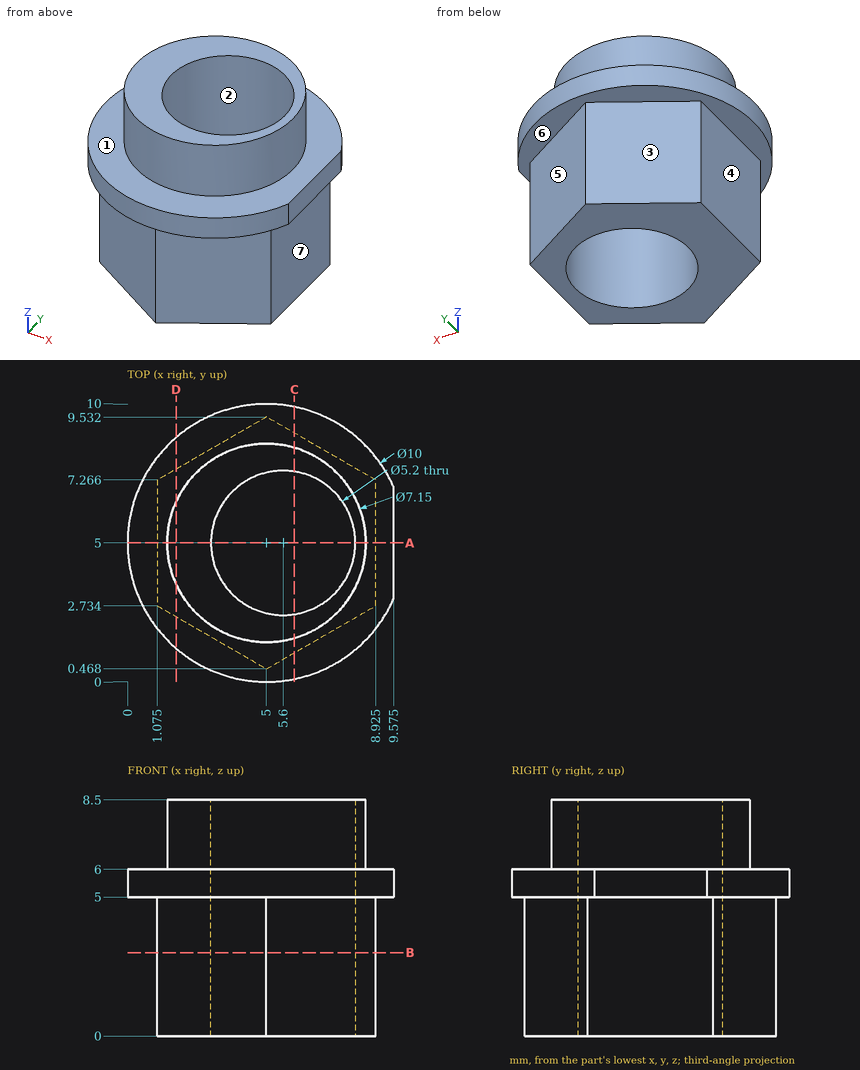
Check sheet for the drawn part. Datum: minimum x, y, z corner. Units: mm. A direction names the side the tool comes from. Round coordinates to 2 decimals unless told otherwise and drop trailing zeros. Order: outer loops, then holes, each group sorted by start corner. A loop starts at its lowest first (then second) coordinate and runs counter-clockwise, first axis right, second up. Notation, with made-up numbers: (36, 49) -> (41, 49) arc R18 cw to (41, 64) -> close; hole circle Ø6 at (78, 45). An arc over 180 degrees is marked (long way). Return JSON: item names as keys, results as strings. Group by question number.
Q1. Section check D-D, the plane x = 1.75. Record the boundary of the cut face in (y, z), plus the area to 3 significant figures.
Q2. Material ranges on probe 1 along Z at (x, y) = (8.5, 6.75); probe 2 along Y at (x, z) = (6, 8.25); probe 3 along X at (y, z) = (6.25, 2.5) (1 decimal), recorded low to high. Write a range as from..to.
Q3. Section check B-B, the plane z = 3. Record the boundary of the cut face in (x, y) (1 decimal), plus the area to 3 significant figures.
Q4. Tool access check on the marked faces 4, 5, 6 and 7. Record the directions out of +Z, -Z, +X, -X, +Y, -Y that give a thin tool (end or side, any length) a straight path to the whole face; none if there is none.
Q5. Section check C-C, the plane x = 6. Record the boundary of the cut face in (y, z) (1 decimal).
Q6. Release check for a two-part mould opening along Y. For the marked faces 1, 2 and 3 record: released by +Y, released by -Y, zero draft, split by the parting line, or undercut.
Q7. Gauge pin test, flat ends, axial feed: pin 1 (1.5 mm diameter, centred on y = 7, z = 2.5, fed in from +X) (3 decimals); pin 2 (5 mm diameter, centred on x = 1, z = 2, fed in from +Y); pin 3 (3.5 mm diameter, centred on y = 6, z = 1.5, fed in from -X) (3 decimals). Record the tip position at first contact, or that the pin passes through.
Q8. Section check A-A, the plane y = 5. Record the boundary of the cut face in (x, z) (3 decimals).
Numbers:
{
 "1": {"outline": "(1.2, 5) -> (2.34, 5) -> (2.34, 0) -> (7.66, 0) -> (7.66, 5) -> (8.8, 5) -> (8.8, 6) -> (6.49, 6) -> (6.49, 8.5) -> (3.51, 8.5) -> (3.51, 6) -> (1.2, 6) -> close", "area": "41.6 mm^2"},
 "2": {"probe 1": "0..6", "probe 2": "1.57..2.43, 7.57..8.43", "probe 3": "1.1..3.3, 7.9..8.9"},
 "3": {"outline": "(1.1, 2.7) -> (5, 0.5) -> (8.9, 2.7) -> (8.9, 7.3) -> (5, 9.5) -> (1.1, 7.3) -> close; hole circle Ø5.2 at (5.6, 5)", "area": "32.1 mm^2"},
 "4": {"face 4": "-Z, -X, +Y, -Y", "face 5": "-Z, +X, +Y", "face 6": "-Z", "face 7": "-Z, +X, +Y, -Y"},
 "5": {"outline": "(0.1, 5) -> (1, 5) -> (1, 0) -> (2.4, 0) -> (2.4, 8.5) -> (1.6, 8.5) -> (1.6, 6) -> (0.1, 6) -> close; (7.6, 0) -> (9, 0) -> (9, 5) -> (9.9, 5) -> (9.9, 6) -> (8.4, 6) -> (8.4, 8.5) -> (7.6, 8.5) -> close"},
 "6": {"face 1": "zero draft", "face 2": "undercut", "face 3": "released by +Y"},
 "7": {"pin 1": "x = 8.925", "pin 2": "y = 8.67", "pin 3": "x = 1.075"},
 "8": {"outline": "(0, 5) -> (1.075, 5) -> (1.075, 0) -> (3, 0) -> (3, 8.5) -> (1.425, 8.5) -> (1.425, 6) -> (0, 6) -> close; (8.2, 0) -> (8.925, 0) -> (8.925, 5) -> (9.575, 5) -> (9.575, 6) -> (8.575, 6) -> (8.575, 8.5) -> (8.2, 8.5) -> close"}
}
